Source: three-view drawing plus pictorial views. Frame: mm from the lowest corner of the part. Give positions to 0.01 mm unless a question says otherwise; leave off trailing zeros. Loops run counter-clockwise (first coordinate to the right, second up) from the corner with the lowest first, then second, coordinate; pieces in that order, holes last. Notation, with made-up numbers: (77.5, 65.5) - (118.5, 65.5) arc R32 cw to (118.5, 94.5) - close; hole circle Ø7 at (75.25, 18.25). An arc over 180 degrees is marked (long way). One line per item, written item: value.
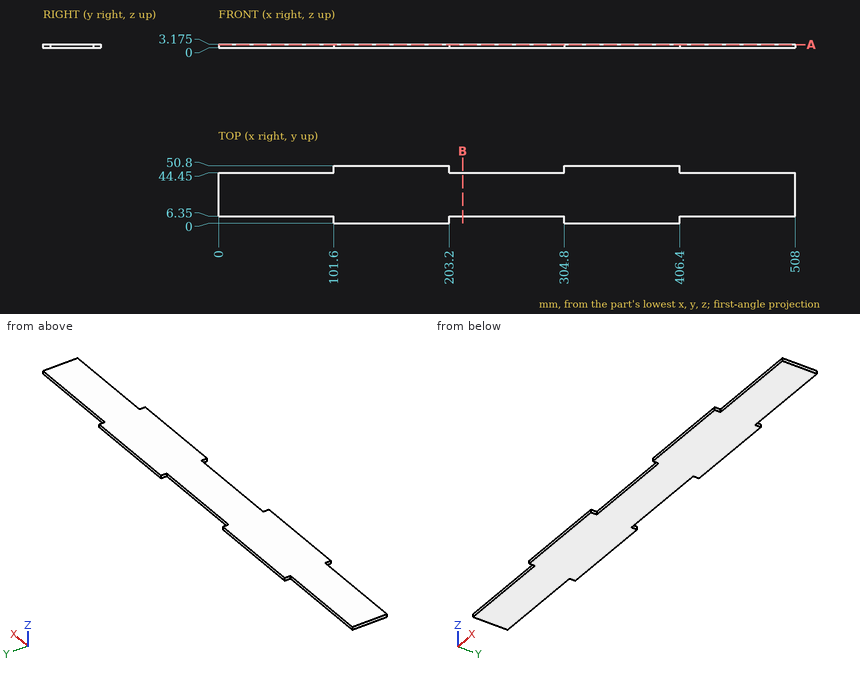
Item 1: Section B-B, the plane x = 215. Output: boundary loops of the cut face in (y, z) (3 decimals), and give its area (3 significant figures).
Verdict:
outline: (6.35, 0) - (44.45, 0) - (44.45, 3.175) - (6.35, 3.175) - close
area: 121 mm^2
Item 2: Section A-A, the plane z = 2.6. Output: boundary loops of the cut face in (x, y).
Verdict:
outline: (0, 6.35) - (101.6, 6.35) - (101.6, 0) - (203.2, 0) - (203.2, 6.35) - (304.8, 6.35) - (304.8, 0) - (406.4, 0) - (406.4, 6.35) - (508, 6.35) - (508, 44.45) - (406.4, 44.45) - (406.4, 50.8) - (304.8, 50.8) - (304.8, 44.45) - (203.2, 44.45) - (203.2, 50.8) - (101.6, 50.8) - (101.6, 44.45) - (0, 44.45) - close
Item 3: Pin query (flat end, axial travel): P1, Ø1, axis at y = 47.5, z = 2, coming from the -X side; P2, Ø1.6, axis at y = 46, z = 1.5, coming from the +X side; P3, Ø1, axis at x = 50.5, z = 1.5, coming from the -Y side. Return the tip coordinate at first contact, or that it passes through.
Verdict:
P1: stops at x = 101.6
P2: stops at x = 406.4
P3: stops at y = 6.35
Item 4: Material intervals for L1, parallel to X at y = 46, z = 1.35; L2, parallel to Y at x = 480.5, z = 2.75, sorted ascending.
Verdict:
L1: x = 101.6 to 203.2, 304.8 to 406.4
L2: y = 6.35 to 44.45
